Autodesk Fusion 360 part; units mm, degrees
sketch "Sketch1" plane through (0, 0, 0) normal (0, 0, 1) x (1, 0, 0)
  line L0 (-78.198, 0.5) -> (78.198, 0.5)
  line L1 (78.198, 0.5) -> (78.198, -0.5)
  line L2 (78.198, -0.5) -> (-78.198, -0.5)
  line L3 (-78.198, -0.5) -> (-78.198, 0.5)
  line L4 (-78.198, 0.5) -> (78.198, -0.5) construction
  line L5 (78.198, 0.5) -> (-78.198, -0.5) construction
  line L6 (-67.4715, -39.532) -> (-67.9715, -38.666)
  line L7 (-67.9715, -38.666) -> (67.9715, 38.666) construction
  line L8 (67.4715, 39.532) -> (67.9715, 38.666)
  line L9 (67.9715, 38.666) -> (-67.4715, -39.532)
  line L10 (-67.9715, -38.666) -> (67.4715, 39.532)
  line L11 (67.4715, 39.532) -> (-67.4715, -39.532) construction
  line L12 (-38.666, -67.9715) -> (-39.532, -67.4715)
  line L13 (-39.532, -67.4715) -> (39.532, 67.4715) construction
  line L14 (38.666, 67.9715) -> (39.532, 67.4715)
  line L15 (39.532, 67.4715) -> (-38.666, -67.9715)
  line L16 (-39.532, -67.4715) -> (38.666, 67.9715)
  line L17 (38.666, 67.9715) -> (-38.666, -67.9715) construction
  line L18 (0.5, -78.198) -> (-0.5, -78.198)
  line L19 (-0.5, -78.198) -> (0.5, 78.198) construction
  line L20 (-0.5, 78.198) -> (0.5, 78.198)
  line L21 (0.5, 78.198) -> (0.5, -78.198)
  line L22 (-0.5, -78.198) -> (-0.5, 78.198)
  line L23 (-0.5, 78.198) -> (0.5, -78.198) construction
  line L24 (39.532, -67.4715) -> (38.666, -67.9715)
  line L25 (38.666, -67.9715) -> (-38.666, 67.9715) construction
  line L26 (-39.532, 67.4715) -> (-38.666, 67.9715)
  line L27 (-38.666, 67.9715) -> (39.532, -67.4715)
  line L28 (38.666, -67.9715) -> (-39.532, 67.4715)
  line L29 (-39.532, 67.4715) -> (39.532, -67.4715) construction
  line L30 (67.9715, -38.666) -> (67.4715, -39.532)
  line L31 (67.4715, -39.532) -> (-67.4715, 39.532) construction
  line L32 (-67.9715, 38.666) -> (-67.4715, 39.532)
  line L33 (-67.4715, 39.532) -> (67.9715, -38.666)
  line L34 (67.4715, -39.532) -> (-67.9715, 38.666)
  line L35 (-67.9715, 38.666) -> (67.9715, -38.666) construction
  line L36 (78.198, 0.5) -> (78.198, -0.5)
  line L37 (78.198, -0.5) -> (-78.198, 0.5) construction
  line L38 (-78.198, -0.5) -> (-78.198, 0.5)
  line L39 (-78.198, 0.5) -> (78.198, 0.5)
  line L40 (78.198, -0.5) -> (-78.198, -0.5)
  line L41 (-78.198, -0.5) -> (78.198, 0.5) construction
  line L42 (67.4715, 39.532) -> (67.9715, 38.666)
  line L43 (67.9715, 38.666) -> (-67.9715, -38.666) construction
  line L44 (-67.4715, -39.532) -> (-67.9715, -38.666)
  line L45 (-67.9715, -38.666) -> (67.4715, 39.532)
  line L46 (67.9715, 38.666) -> (-67.4715, -39.532)
  line L47 (-67.4715, -39.532) -> (67.4715, 39.532) construction
  line L48 (38.666, 67.9715) -> (39.532, 67.4715)
  line L49 (39.532, 67.4715) -> (-39.532, -67.4715) construction
  line L50 (-38.666, -67.9715) -> (-39.532, -67.4715)
  line L51 (-39.532, -67.4715) -> (38.666, 67.9715)
  line L52 (39.532, 67.4715) -> (-38.666, -67.9715)
  line L53 (-38.666, -67.9715) -> (38.666, 67.9715) construction
  line L54 (-0.5, 78.198) -> (0.5, 78.198)
  line L55 (0.5, 78.198) -> (-0.5, -78.198) construction
  line L56 (0.5, -78.198) -> (-0.5, -78.198)
  line L57 (-0.5, -78.198) -> (-0.5, 78.198)
  line L58 (0.5, 78.198) -> (0.5, -78.198)
  line L59 (0.5, -78.198) -> (-0.5, 78.198) construction
  line L60 (-39.532, 67.4715) -> (-38.666, 67.9715)
  line L61 (-38.666, 67.9715) -> (38.666, -67.9715) construction
  line L62 (39.532, -67.4715) -> (38.666, -67.9715)
  line L63 (38.666, -67.9715) -> (-39.532, 67.4715)
  line L64 (-38.666, 67.9715) -> (39.532, -67.4715)
  line L65 (39.532, -67.4715) -> (-39.532, 67.4715) construction
  line L66 (-67.9715, 38.666) -> (-67.4715, 39.532)
  line L67 (-67.4715, 39.532) -> (67.4715, -39.532) construction
  line L68 (67.9715, -38.666) -> (67.4715, -39.532)
  line L69 (67.4715, -39.532) -> (-67.9715, 38.666)
  line L70 (-67.4715, 39.532) -> (67.9715, -38.666)
  line L71 (67.9715, -38.666) -> (-67.9715, 38.666) construction
  dimension "d1" = 1
  dimension "d3" = 360
extrude "Extrude1" add sketch "Sketch1" along normal blind 132.557
Geometry: final body of the model. Coordinates: model frame, mm. A direction names the side the tool comes from. Give positions to 0.01 mm unless a question says otherwise; leave off trailing zeros. Order: outer loops, then holes, each group sorted by start corner. A loop starts at its lowest first (then second) coordinate and runs counter-clockwise, first axis right, second up. Notation, with made-up numbers: (29, -2) -> (47, -2) arc R24 ccw to (47, 37) -> close; hole circle Ø3 at (-38, 9.25). An arc over 180 degrees is marked (long way). Write each question's results on one line, items separated by ' | '.
1) First-contact query: pin 1 Ø3 at (y, z) = (-24, 98) entering from +X; pin 2 Ø10 at (x, z) = (10, 100.5) entering from -Y; pin 3 Ø1 at (y, z) = (39.5, 84.5) entering from -X. Flat tips, straight axial feed; report the tip coordinate or a pass-through.
Geometry says:
pin 1: stops at x = 45.17 | pin 2: stops at y = -26.98 | pin 3: stops at x = -67.78
2) Line query: line 1 along Y through (x, z) = (16, 85); line 2 along Y through (x, z) = (51, 98); line 3 along Y through (x, z) = (21.5, 19). Output: solid intervals per line, ascending.
Geometry says:
line 1: y = -28.71 to -26.71, -9.81 to -8.66, -0.5 to 0.5, 8.66 to 9.81, 26.71 to 28.71 | line 2: y = -30.02 to -28.87, -0.5 to 0.5, 28.87 to 30.02 | line 3: y = -38.24 to -36.24, -12.99 to -11.84, -0.5 to 0.5, 11.84 to 12.99, 36.24 to 38.24
3) Draft query along Y for faces 5 (the face through (-33.956, -20.182, 65.351)), 6 (the face through (-39, -0.5, 65)), 7 (the face through (-19.32, -34.46, 65.35)), 8 (the face through (-19.85, 35.38, 65.35)). Return one class per face: released by +Y, released by -Y, zero draft, split by the parting line, or undercut.
Geometry says:
face 5: undercut | face 6: undercut | face 7: released by -Y | face 8: released by +Y
4) Cut plane C-C (x = 51). Output: boundary loops of the cut face in (y, z), and give its area (3 significant figures).
Geometry says:
outline: (-30.02, 0) -> (-28.87, 0) -> (-28.87, 132.56) -> (-30.02, 132.56) -> close; (-0.5, 0) -> (0.5, 0) -> (0.5, 132.56) -> (-0.5, 132.56) -> close; (28.87, 0) -> (30.02, 0) -> (30.02, 132.56) -> (28.87, 132.56) -> close | area: 439 mm²
5) Cut plane A-A (y = 25.5). Output: boundary loops of the cut face in (x, z).
Geometry says:
outline: (-45.17, 0) -> (-43.17, 0) -> (-43.17, 132.56) -> (-45.17, 132.56) -> close; (-15.3, 0) -> (-14.15, 0) -> (-14.15, 132.56) -> (-15.3, 132.56) -> close; (-0.5, 0) -> (0.5, 0) -> (0.5, 132.56) -> (-0.5, 132.56) -> close; (14.15, 0) -> (15.3, 0) -> (15.3, 132.56) -> (14.15, 132.56) -> close; (43.17, 0) -> (45.17, 0) -> (45.17, 132.56) -> (43.17, 132.56) -> close
6) Cut plane B-B (x = -21). Output: boundary loops of the cut face in (y, z).
Geometry says:
outline: (-37.37, 0) -> (-35.37, 0) -> (-35.37, 132.56) -> (-37.37, 132.56) -> close; (-12.7, 0) -> (-11.55, 0) -> (-11.55, 132.56) -> (-12.7, 132.56) -> close; (-0.5, 0) -> (0.5, 0) -> (0.5, 132.56) -> (-0.5, 132.56) -> close; (11.55, 0) -> (12.7, 0) -> (12.7, 132.56) -> (11.55, 132.56) -> close; (35.37, 0) -> (37.37, 0) -> (37.37, 132.56) -> (35.37, 132.56) -> close
7) Set-up query: faces 1 (the face through (19.85, -35.38, 65.35)), 2 (the face through (-34.881, 20.716, 65.351)), 3 (the face through (0.5, 41, 65)), 4 (the face through (35.38, 19.85, 65.35)). Return all of +Z, -Z, +X, -X, +Y, -Y with unobstructed straight access to the full face (end or side cutting, diameter ignored); none if empty.
Geometry says:
face 1: +Z, -Z, -Y | face 2: +Z, -Z | face 3: +Z, -Z, +Y | face 4: +Z, -Z, +X
